from build123d import *

# Parameters (mm, degrees)
F0_R             = 12.5
F1_DEPTH         = 2
F2_R             = 6
F3_DEPTH         = 0.8
F4_R             = 4
F5_DEPTH         = 4
F6_R             = 2
F7_DEPTH         = 6.8
F8_R             = 4.5
F8_R_2           = 3.25
F9_DEPTH         = 3
F10_W            = 8.2
F10_H            = 3
F11_DEPTH        = 0.8
F11_DEPTH_BACK   = 0.8
F11_COPIES_COUNT = 6


# Not quite as in the source:
# - a pattern or mirror of a feature is missing from the dataset's text; its kind, count and spacing are read off the source's solid


with BuildPart() as f1:
    # F0 (on Top) → F1 (new body)
    with BuildSketch(Plane.XY):
        Circle(F0_R)
    extrude(amount=F1_DEPTH)

    # F2 (on face) → F3 (join)
    with BuildSketch(Plane.XY.offset(2)):
        Circle(F2_R)
    extrude(amount=F3_DEPTH)

    # F4 (on face) → F5 (join)
    with BuildSketch(Plane.XY.offset(2.8)):
        Circle(F4_R)
    extrude(amount=F5_DEPTH)

    # F6 (on face) → F7 (cut, through all)
    with BuildSketch(Plane.XY.offset(6.8)):
        Circle(F6_R)
    extrude(amount=-F7_DEPTH, mode=Mode.SUBTRACT)

    # F8 (on face) → F9 (join)
    with BuildSketch(Plane(origin=(0, 0, 0), x_dir=(1, 0, 0), z_dir=(0, 0, -1))):
        Circle(F8_R)
        Circle(F8_R_2, mode=Mode.SUBTRACT)
    extrude(amount=F9_DEPTH)

    # F10 (on Front) → F11 (join, two sides)
    with BuildSketch(Plane.XZ) as f11_sk:
        with Locations((-8.4, -1.5)):
            Rectangle(F10_W, F10_H)
    f11 = extrude(amount=F11_DEPTH) + extrude(f11_sk.sketch, amount=-F11_DEPTH_BACK)

    # F11_copies: F11 ×6 about axis
    f11_copies_axis = Axis((0, 0, 0), (0, 0, 1))
    for i in range(1, F11_COPIES_COUNT):
        add(f11.rotate(f11_copies_axis, i * 360 / F11_COPIES_COUNT))


solid = f1.part
Work out the finished part from the listing and answer in its coordinate system (mm). A direction names the side the tool comes from. Round coordinates to 2 decimals unless told otherwise and drop trailing zeros. Loops run counter-clockwise (first coordinate to the right, second up) from the corner with the lowest first, then second, coordinate; pieces in that order, holes last. Notation, with made-up numbers: (63.25, 60.25) - (79.25, 60.25) arc R26 ccw to (79.25, 97.25) - close; hole circle Ø10 at (16, 11.5). An arc over 180 degrees is marked (long way). Use one line per item in the form item = value. Start each with the question number.
(1) Determine the mould class of faces 5 (the face through (-6.24, 10.83, -1.52)), 6 (the face through (12.5, 0, -2)), 7 (the face through (4.953, 6.979, -1.479)) for opening direction Y: +Y half, -Y half, draft (parallel to the pull), parting line (faces both ways), or undercut.
(2) Find section A-A on x = 0. Determine the outline of the cut face in (y, z), and give its area (3 significant figures).
(3) Find section B-B on z = -2. Determine the outline of the cut face in (x, y), and give its area (3 significant figures).
(4) Find section D-D on x = 10.75. Determine the outline of the cut face in (y, z), and give its area (3 significant figures).
(5) Find section C-C on y = 7.5. Determine the outline of the cut face in (x, z), and give its area (3 significant figures).
(6) Flat-ended cylindrical pins translate along their axes: P1, Ø1.5, axis at x = 7.5, z = -1, coming from the +Y side; P2, Ø6, axis at x = -7.5, y = -4, coming from the +Z side; P3, Ø2, axis at x = 3.5, z = 3.5, coming from the -Y side. Find the tip coordinate at first contact, or state that the pin passes through.
(7) Which of the six approach directions +Z, -Z, +X, -X, +Y, -Y give full straight-line access (tool end or side, diameter ignored) to faces 1 (the face through (-3.886, -2.269, -1.479)), 2 (the face through (1, -2, 0)), 3 (the face through (-5.994, 0.264, 2.394)), 4 (the face through (4.953, -6.979, -1.479))?
(8) Consider line 1 (Y direction, x = 0, z = 1.5); line 2 (X direction, y = 0, z = -1.95); line 3 (Y direction, x = -5.5, z = -1.25). Determine where each line is inside the solid, lowest interval first.
Answer list:
q1.face_5 = +Y half
q1.face_6 = draft
q1.face_7 = undercut
q2.outline = (-12.5, 0) - (-4.5, 0) - (-4.5, -3) - (-3.25, -3) - (-3.25, 0) - (-2, 0) - (-2, 6.8) - (-4, 6.8) - (-4, 2.8) - (-6, 2.8) - (-6, 2) - (-12.5, 2) - close; (2, 0) - (3.25, 0) - (3.25, -3) - (4.5, -3) - (4.5, 0) - (12.5, 0) - (12.5, 2) - (6, 2) - (6, 2.8) - (4, 2.8) - (4, 6.8) - (2, 6.8) - close
q2.area = 71.9 mm^2
q3.outline = (-12.5, -0.8) - (-4.43, -0.8) arc R4.5 ccw to (-2.91, -3.44) - (-6.94, -10.43) - (-5.56, -11.23) - (-1.52, -4.24) arc R4.5 ccw to (1.52, -4.24) - (5.56, -11.23) - (6.94, -10.43) - (2.91, -3.44) arc R4.5 ccw to (4.43, -0.8) - (12.5, -0.8) - (12.5, 0.8) - (4.43, 0.8) arc R4.5 ccw to (2.91, 3.44) - (6.94, 10.43) - (5.56, 11.23) - (1.52, 4.24) arc R4.5 ccw to (-1.52, 4.24) - (-5.56, 11.23) - (-6.94, 10.43) - (-2.91, 3.44) arc R4.5 ccw to (-4.43, 0.8) - (-12.5, 0.8) - close; hole circle Ø6.5 at (0, 0)
q3.area = 107 mm^2
q4.outline = (-6.38, 0) - (-0.8, 0) - (-0.8, -3) - (0.8, -3) - (0.8, 0) - (6.38, 0) - (6.38, 2) - (-6.38, 2) - close
q4.area = 30.3 mm^2
q5.outline = (-10, 0) - (-5.25, 0) - (-5.25, -3) - (-3.41, -3) - (-3.41, 0) - (3.41, 0) - (3.41, -3) - (5.25, -3) - (5.25, 0) - (10, 0) - (10, 2) - (-10, 2) - close
q5.area = 51.1 mm^2
q6.P1 = 10.54
q6.P2 = 2.8
q6.P3 = -5.31
q7.face_1 = -Z, -X
q7.face_2 = -Z
q7.face_3 = +Z
q7.face_4 = -Z, +X
q8.line_1 = -12.5 to -2, 2 to 12.5
q8.line_2 = -12.5 to -3.25, 3.25 to 12.5
q8.line_3 = -11.13 to -7.93, -0.8 to 0.8, 7.93 to 11.13
